Could you check a few things on this model? Use its own coordinates, in mm. A direction names the side the tool comes from. Coordinates: 2 decimals unless noted, no trailing zeros. Order: outer loops, then holes, each group sorted by start corner. A loop starts at its lowest first (then second) coordinate and runs counter-clockwise, first axis right, second up. Notation, with made-up numbers: (15, 2) - (19, 2) arc R22 ccw to (19, 11) - close; hole circle Ø4 at (33, 48.25). An arc over 180 degrees is marked (long way). Answer as a JSON object with one key per item and string values. Group by question number.
(1) Imagine slicing it at A-A, the plane z = 0.95. Write out the boundary of the cut face in (x, y).
(2) Imagine slicing it at C-C, the plane y = -35. Write out the boundary of the cut face in (x, z).
(3) Imagine slicing it at B-B, the plane x = 0. Write out the boundary of the cut face in (y, z).
(4) Which directions (+Z, -Z, +X, -X, +Y, -Y) give clear straight access to the entire face, cutting with the end or side of a thin tool? Please do faces 1 (the flat face through (0, -18, 1)), 2 (the flat face through (33.976, 1.459, 1.479)).
(5) We'd pull the mould along Y, two halves only. Please class faces 3 (the cylindrical face through (-0.06, -43.75, 1.52)), 4 (the cylindrical face through (-42.92, 30.41, 1.52)), 5 (the flat face through (-1, 21, 0)), 6 (the flat face through (-18, 0, 1)): pulls with the +Y half, pulls with the -Y half, needs draft (parallel to the pull), parting line crosses it, or undercut.
(6) Please list where these lines run through material, in increasing order: probe 1 along Y at (x, z) = (0, 2.15); probe 2 along Y at (x, z) = (-1, 1.65); probe 3 along X at (y, z) = (28.5, 2.55).
(7) Will these pins go through, and if not, where does the flat tip stop? P1, Ø1.5, axis at y = -3, z = 1.5, coming from the -X side; P2, Ø0.9, axis at x = 5.5, z = 2, coming from the -Y side; P3, Ø8, axis at x = 35, y = 25, coming from the +Z side.
(8) Imagine slicing it at D-D, the plane x = -10. Write out the boundary of the cut face in (y, z), and give its area (3 significant figures).
Autodesk Inventor part; units mm, degrees
ref_plane "YZ Plane" through (0, 0, 0) normal (1, 0, 0) x (0, 1, 0)
ref_plane "XZ Plane" through (0, 0, 0) normal (0, 1, 0) x (-1, 0, 0)
ref_plane "XY Plane" through (0, 0, 0) normal (0, 0, 1) x (1, 0, 0)
sketch "Sketch6" plane through (0, 0, 0) normal (0, 0, 1) x (1, 0, 0)
  line L0 (18, 18) -> (-18, 18)
  line L1 (-18, 18) -> (-18, -18)
  line L2 (-18, -18) -> (18, -18)
  line L3 (18, -18) -> (18, 18)
  line L4 (18, 18) -> (-18, -18) construction
  circle A0 centre (0, -35) radius 5.05
  circle A1 centre (35, 25) radius 5.05
  circle A2 centre (-35, 25) radius 5.05
  line L5 (35, 25) -> (-35, 25) construction
  line L6 (-35, 25) -> (0, -35) construction
  line L7 (0, -35) -> (35, 25) construction
  line L8 (0, 18) -> (0, -18) construction
  line L9 (-46.936, 33) -> (46.936, 33)
  line L10 (-18, 18) -> (23.6569, -23.6569) construction
  line L11 (18, 18) -> (-23.6569, -23.6569) construction
  line L12 (46.936, 33) -> (23.6569, -23.6569)
  line L13 (23.6569, -23.6569) -> (0, -46.0053)
  line L14 (0, -46.0053) -> (-23.6569, -23.6569)
  line L15 (-46.936, 33) -> (-23.6569, -23.6569)
  line L16 (-35, 25) -> (-42.3997, 21.9596) construction
  line L17 (0, -35) -> (-5.4937, -40.8154) construction
  point P0 (0, 0)
  point P1 (0, 0)
  point P2 (60, 0)
  point P3 (0, 33)
  point P4 (0, 0)
  dimension "d30" = 36
  dimension "d31" = 36
  dimension "d33" = 10.1
  dimension "d37" = 69.4622
  dimension "d52" = 70
  dimension "d53" = 8
  dimension "d54" = 25
  dimension "d57" = 8
  dimension "d59" = 8
  dimension "d60" = 93.872
  dimension "d61" = 60
  dimension "d62" = 8
  dimension "d63" = 8
extrude "Plate3" add sketch "Sketch6" along normal blind 3
fillet "Corner Round2" radius 6 5 edges at (-46.936, 33, 1.5) (46.936, 33, 1.5) (0, -46.0053, 1.5) (-23.6569, -23.6569, 1.5) (23.6569, -23.6569, 1.5)
equation "\"d41\" = Thickness"
equation "\"BendReliefWidth\" = Thickness"
equation "\"BendReliefDepth\" = 0.5 * Thickness"
equation "\"CornerReliefSize\" = 4 * Thickness"
equation "\"MinimumRemnant\" = 2 * Thickness"
equation "\"TransitionRadius\" = BendRadius"
equation "\"JacobiRadiusSize\" = BendRadius"
equation "\"GapSize\" = Thickness"
properties part number "DS-B-501 beam flange" material "Stainless Steel"
Result set:
{
 "1": {"outline": "(-43.53, 24.72) - (-24.15, -22.46) arc R6 ccw to (-22.72, -24.54) - (-4.12, -42.11) arc R6 ccw to (4.12, -42.11) - (22.72, -24.54) arc R6 ccw to (24.15, -22.46) - (43.53, 24.72) arc R6 ccw to (37.98, 33) - (-37.98, 33) arc R6 ccw to start; hole circle Ø10.1 at (-35, 25); hole (-18, -18) - (18, -18) - (18, 18) - (-18, 18) - close; hole circle Ø10.1 at (0, -35); hole circle Ø10.1 at (35, 25)"},
 "2": {"outline": "(-11.65, 0) - (-5.05, 0) - (-5.05, 3) - (-11.65, 3) - close; (5.05, 0) - (11.65, 0) - (11.65, 3) - (5.05, 3) - close"},
 "3": {"outline": "(-43.75, 0) - (-40.05, 0) - (-40.05, 3) - (-43.75, 3) - close; (-29.95, 0) - (-18, 0) - (-18, 3) - (-29.95, 3) - close; (18, 0) - (33, 0) - (33, 3) - (18, 3) - close"},
 "4": {"face 1": "+Z, -Z", "face 2": "+Z, -Z, +X, -Y"},
 "5": {"face 3": "pulls with the -Y half", "face 4": "parting line crosses it", "face 5": "needs draft", "face 6": "undercut"},
 "6": {"probe 1": "y = -43.75 to -40.05, -29.95 to -18, 18 to 33", "probe 2": "y = -43.67 to -39.95, -30.05 to -18, 18 to 33", "probe 3": "x = -43.79 to -38.64, -31.36 to 31.36, 38.64 to 43.79"},
 "7": {"P1": "stops at x = -32.45", "P2": "stops at y = -41.23", "P3": "passes through"},
 "8": {"outline": "(-36.56, 0) - (-18, 0) - (-18, 3) - (-36.56, 3) - close; (18, 0) - (33, 0) - (33, 3) - (18, 3) - close", "area": "101 mm^2"}
}
